Verification items for the finished model (mm, model axes). Face numbers are marked on the shaded views. A direction names the side the tool comes from. Round coordinates to 2 decimals unless told otherwise and drop trailing zeros. Order: outer loops, then holes, each group sorted by start corner. A loop starts at its lowest first (then second) coordinate and runs counter-clockwise, first axis right, second up. Notation, with made-up numbers: (13, -21) -> (17, -21) arc R17 ccw to (17, -12) -> close; hole circle Ø3 at (17, -6). An arc over 180 degrees is marked (long way). Put each result on its own line as item: value.
from build123d import *

# Parameters (mm, degrees)
F0_W     = 304.8
F0_H     = 228.6
F0_W_2   = 292.1
F0_H_2   = 127
F1_DEPTH = 5
F2_W     = 304.8
F2_H     = 228.6
F3_DEPTH = 203.2
F4_W     = 228.6
F4_H     = 76.2
F5_DEPTH = 228.601
F6_W     = 152.4
F6_H     = 76.2
F7_DEPTH = 304.801
F8_R     = 50.8
F9_R     = 19.05
F10_R    = 12.7


with BuildPart() as f1:
    # F0 (on Top) → F1 (new body)
    with BuildSketch(Plane.XY):
        Rectangle(F0_W, F0_H)
        Rectangle(F0_W_2, F0_H_2, mode=Mode.SUBTRACT)
    extrude(amount=F1_DEPTH)

    # F2 (on face) → F3 (join)
    with BuildSketch(Plane.XY.offset(5)):
        Rectangle(F2_W, F2_H)
        Polygon((-146.0499983072, 63.5), (-146.0499983072, 107.9499983072), (146.0499983072, 107.9499983072), (146.0499983072, 63.5), (146.0499983072, -63.5), (146.0499983072, -107.9499983072), (-146.0499983072, -107.9499983072), (-146.0499983072, -63.5), align=None, mode=Mode.SUBTRACT)
    extrude(amount=F3_DEPTH)

    # F4 (on face) → F5 (cut, through all)
    with BuildSketch(Plane.XZ.offset(114.3)):
        with Locations((0, 170.1)):
            Rectangle(F4_W, F4_H)
    extrude(amount=-F5_DEPTH, mode=Mode.SUBTRACT)

    # F6 (on face) → F7 (cut, through all)
    with BuildSketch(Plane.YZ.offset(152.4)):
        with Locations((0, 170.1)):
            Rectangle(F6_W, F6_H)
    extrude(amount=-F7_DEPTH, mode=Mode.SUBTRACT)

    # F8
    f8_edges = [f1.edges().sort_by_distance(p)[0] for p in [
        (-114.3, -111.124999, 132),
        (-149.224999, 76.2, 132),
        (-114.3, 111.124999, 132),
        (-149.224999, -76.2, 132),
        (114.3, 111.124999, 132),
        (149.224999, -76.2, 132),
        (114.3, -111.124999, 132),
        (149.224999, 76.2, 132),
    ]]
    fillet(f8_edges, radius=F8_R)

    # F9
    f9_edges = [f1.edges().sort_by_distance(p)[0] for p in [
        (149.224999, 76.2, 208.2),
        (114.3, 111.124999, 208.2),
        (-114.3, 111.124999, 208.2),
        (-149.224999, 76.2, 208.2),
        (-149.224999, -76.2, 208.2),
        (-114.3, -111.124999, 208.2),
        (114.3, -111.124999, 208.2),
        (149.224999, -76.2, 208.2),
    ]]
    fillet(f9_edges, radius=F9_R)

    # F10
    f10_edges = [f1.edges().sort_by_distance(p)[0] for p in [
        (152.4, -114.3, 104.1),
        (146.049998, -107.949998, 106.6),
        (-152.4, -114.3, 104.1),
        (146.049998, 107.949998, 106.6),
        (-146.049998, 107.949998, 106.6),
        (-146.049998, -107.949998, 106.6),
        (-152.4, 114.3, 104.1),
        (152.4, 114.3, 104.1),
    ]]
    fillet(f10_edges, radius=F10_R)


solid = f1.part
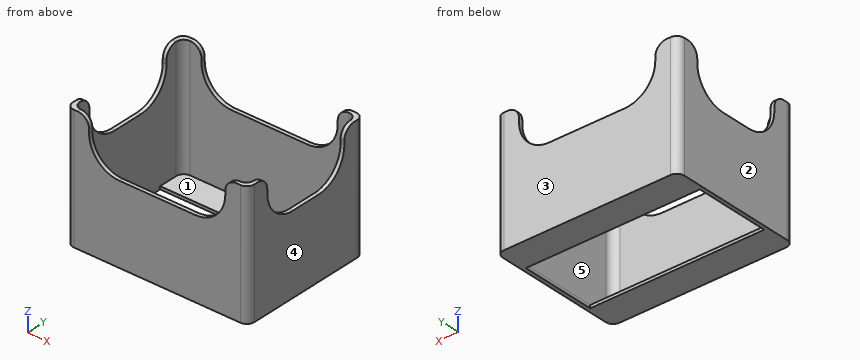
Item 1: Section check B-B on z = 45.5. Record the boundary of the cut face in (x, y).
Check sheet entries:
outline: (-152.4, -101.6) arc R12.7 ccw to (-139.7, -114.3) -> (139.7, -114.3) arc R12.7 ccw to (152.4, -101.6) -> (152.4, 101.6) arc R12.7 ccw to (139.7, 114.3) -> (-139.7, 114.3) arc R12.7 ccw to (-152.4, 101.6) -> close; hole (-146.05, -95.25) arc R12.7 ccw to (-133.35, -107.95) -> (133.35, -107.95) arc R12.7 ccw to (146.05, -95.25) -> (146.05, 95.25) arc R12.7 ccw to (133.35, 107.95) -> (-133.35, 107.95) arc R12.7 ccw to (-146.05, 95.25) -> close
Item 2: Gauge pin test, flat ends, axial feed: pin 1 Ø1.9 at (x, z) = (149.5, 185.5) entering from +Y; pin 2 Ø5 at (x, z) = (-148.5, 187) entering from -Y; pin 3 Ø4 at (x, y) = (1.5, 66.5) entering from +Z; pin 4 Ø12 at (x, y) = (-91.5, -54) entering from +Z. Record the tip position at first contact, or that the pin passes through.
Check sheet entries:
pin 1: stops at y = 110.71
pin 2: stops at y = -112.63
pin 3: stops at z = 5
pin 4: passes through
Item 3: Release check for a two-part mould opening along X. For the marked faces 1, 2 and 3 record: +X half, -X half, draft (parallel to the pull), parting line (faces both ways), or undercut.
Check sheet entries:
face 1: undercut
face 2: -X half
face 3: draft
Item 4: Tool access check on the marked faces 4 and 5. Record the directions out of +Z, -Z, +X, -X, +Y, -Y that give a thin tool (end or side, any length) a straight path to the whole face; none if there is none.
Check sheet entries:
face 4: +Z, -Z, +X, +Y, -Y
face 5: +Z
Item 5: Section check D-D on z = 177. State how many separate pieces and enclosed holes the cut face has, then the cut area to 3 significant figures.
Check sheet entries:
separate pieces: 4
enclosed holes: 0
area: 1,790 mm^2
Item 6: Material ranges on L1, parallel to X at y = -95.5, z = 85; L2, parallel to Y at x = 127, z = 34; L3, parallel to Z at x = 103.5, y = -95.5, recorded low to high. Write a range as [from, to].
Check sheet entries:
L1: x = [-152.4, -146.05], [146.05, 152.4]
L2: y = [-114.3, -107.95], [107.95, 114.3]
L3: z = [0, 5]
Item 7: Section check A-A on x = -40. Record the boundary of the cut face in (y, z).
Check sheet entries:
outline: (-114.3, 0) -> (-63.5, 0) -> (-63.5, 5) -> (-107.95, 5) -> (-107.95, 132) -> (-114.3, 132) -> close; (63.5, 0) -> (114.3, 0) -> (114.3, 132) -> (107.95, 132) -> (107.95, 5) -> (63.5, 5) -> close
